Autodesk Inventor part; units mm, degrees
ref_plane "YZ Plane" through (0, 0, 0) normal (1, 0, 0) x (0, 1, 0)
ref_plane "XZ Plane" through (0, 0, 0) normal (0, 1, 0) x (-1, 0, 0)
ref_plane "XY Plane" through (0, 0, 0) normal (0, 0, 1) x (1, 0, 0)
sketch "Sketch1" plane through (0, 0, 0) normal (0, 1, 0) x (-1, 0, 0)
  line L0 (0, 0) -> (40.2, 0)
  line L1 (40.2, 0) -> (40.2, -155.2)
  line L2 (40.2, -155.2) -> (0, -155.2)
  line L3 (0, -155.2) -> (0, 0)
  line L4 (0, -20) -> (20.2, -20)
  line L5 (20.2, -20) -> (20.2, -135.2)
  line L6 (20.2, -135.2) -> (0, -135.2)
  line L7 (0, -135.2) -> (0, -20)
  line L8 (10.1, -135.2) -> (10.1, -20) construction
  line L9 (20.2, -77.6) -> (0, -77.6) construction
  circle A0 centre (10.1, -77.6) radius 3.5
  line L10 (0, -54.6) -> (20.2, -54.6) construction
  line L11 (20.2, -31.6) -> (0, -31.6) construction
  circle A1 centre (10.1, -54.6) radius 3.5
  circle A2 centre (10.1, -31.6) radius 3.5
  circle A3 centre (10.1, -100.6) radius 3.5
  circle A4 centre (10.1, -123.6) radius 3.5
  line L12 (40.2, -155.2) -> (20.2, -135.2) construction
  line L13 (30.2, -155.2) -> (30.2, 0) construction
  line L14 (20.2, -20) -> (40.2, 0) construction
  circle A5 centre (30.2, -145.2) radius 2.6
  circle A6 centre (30.2, -10) radius 2.6
  circle A7 centre (30.2, -77.6) radius 2.6
  point P0 (0, -135.2)
  dimension "d0" = 115.2
  dimension "d1" = 20.2
  dimension "d2" = 7
  dimension "d3" = 23
  dimension "d4" = 23
  dimension "d11" = 20
  dimension "d12" = 20
  dimension "d13" = 20
  dimension "d14" = 5.2
extrude "Extrusion1" add sketch "Sketch1" along normal blind 12 contours L4 L5 L6 L3
extrude "Extrusion2" add sketch "Sketch1" along normal blind 2 contours A0 | A1 | A2 | A3 | A4
extrude "Extrusion3" add sketch "Sketch1" along normal blind 19 contours L0 L1 L2 L3 L6 L5 L4
equation "\"d1\" = screwTabWidth + tolerance"
equation "\"d2\" = insertDiameter"
equation "\"d11\" = screwTabWidth"
equation "\"d12\" = screwTabWidth"
equation "\"d13\" = screwTabWidth"
equation "\"d14\" = screwDiameter + tolerance"
equation "\"d5\" = insertPadding + insertLength"
equation "\"d7\" = insertPadding"
equation "\"d9\" = insertLength + insertPadding + baseThickness"
equation "\"insertDiameter\" = 7"
equation "\"insertLength\" = 10"
equation "\"insertPadding\" = 2"
equation "\"tolerance\" = 0.2"
equation "\"cellSpacing_1\" = 1"
equation "\"screwDiameter_1\" = 5"
equation "\"baseThickness_1\" = 7"
equation "\"tabThickness_1\" = 0.8"
equation "\"batteryBoxWidth\" = 162"
equation "\"sheetMetalThickness\" = 3.175"
properties part number "CO-1-1-CellSpacerMount"
CAD build for the part. Positions are in the model's coordinates, mm. A direction names the side the tool comes from. Coordinates: 2 decimals unless noted, no trailing zeros. Write each loop counter-clockwise with the first axis right and the second up, starting at its lowest first coordinate (ties: lowest second). Pieces come first, ordered by that corner, then holes. Notation, with made-up numbers: (-16.5, -6) -> (6.5, -6) arc R15 cw to (6.5, 19) -> close; hole circle Ø10 at (81, 68). An arc over 180 degrees is marked (long way). Use CSV: the item, a comma, the result in double quotes. Start each with the question number.
Item 1: Band-saw the part on C-C, the plane x = -30.2. Write the cut outline in (y, z), plus the area to 3 significant figures.
Item 2: Band-saw the part on D-D, the plane z = -54.6. Write the cut outline in (x, y).
Item 3: Band-saw the part on A-A, the plane z = -145.2. Write the cut outline in (x, y).
Item 4: Drop flat-ended pins along their axis: P1, Ø9, axis at x = -10.1, z = -31.6, coming from the +Y side; P2, Ø4, axis at x = -30.2, z = -145.2, coming from the +Y side; P3, Ø4, axis at x = -10.1, z = -100.6, coming from the +Y side; P4, Ø3.5, axis at y = 15, z = -89.5, coming from the +X side. Give the stop position or say it passes through.
Item 5: Tool access for faces 1 (the flat face through (-5, 12, -77)), 2 (the flat face through (-20, 9, -155.2)), 3 (the flat face through (-10, 2, -32)): list every direction of +Z, -Z, +X, -X, +Y, -Y with a clear straight run to the whole face (end or side of a thin tool).
Item 6: Two-plate mould, pull along X, no slides. Class faces 4 (the cylindrical face through (-7.52, 6.93, -125.965)), 5 (the flat face through (0, 7, -79)), 6 (the cylindrical face through (-28.137, 9.367, -76.018)), 7 (the flat face through (-40.2, 9, -77)): +X half, -X half, draft (parallel to the pull), parting line (faces both ways), or undercut.
Item 7: Band-saw the part on B-B, the plane y = 9. Give the number of separate pieces and of enclosed holes in the cut face, plus the area to 3 significant figures.
Item 8: Wall check: probe 1 along Z at (x, y) = (-30.2, 10.5); probe 2 along Z at (x, y) = (-10.1, 4); probe 3 along Z at (x, y) = (-32.5, 13). Give the ranges that are in metal, low to high.
Response values:
1,outline,"(0, -155.2) -> (19, -155.2) -> (19, -147.8) -> (0, -147.8) -> close; (0, -142.6) -> (19, -142.6) -> (19, -80.2) -> (0, -80.2) -> close; (0, -75) -> (19, -75) -> (19, -12.6) -> (0, -12.6) -> close; (0, -7.4) -> (19, -7.4) -> (19, 0) -> (0, 0) -> close"
1,area,"2,650 mm2"
2,outline,"(-40.2, 0) -> (0, 0) -> (0, 12) -> (-6.6, 12) -> (-6.6, 2) -> (-13.6, 2) -> (-13.6, 12) -> (-20.2, 12) -> (-20.2, 19) -> (-40.2, 19) -> close"
3,outline,"(-40.2, 0) -> (-32.8, 0) -> (-32.8, 19) -> (-40.2, 19) -> close; (-27.6, 0) -> (0, 0) -> (0, 19) -> (-27.6, 19) -> close"
4,P1,"stops at y = 12"
4,P2,"passes through"
4,P3,"stops at y = 2"
4,P4,"stops at x = -20.2"
5,face 1,"+X, +Y"
5,face 2,"-Z, +X, -X, +Y, -Y"
5,face 3,"+Y"
6,face 4,"undercut"
6,face 5,"+X half"
6,face 6,"undercut"
6,face 7,"-X half"
7,separate pieces,"1"
7,enclosed holes,"8"
7,area,"5,980 mm2"
8,probe 1,"z = -155.2 to -147.8, -142.6 to -80.2, -75 to -12.6, -7.4 to 0"
8,probe 2,"z = -155.2 to -127.1, -120.1 to -104.1, -97.1 to -81.1, -74.1 to -58.1, -51.1 to -35.1, -28.1 to 0"
8,probe 3,"z = -155.2 to -146.41, -143.99 to -78.81, -76.39 to -11.21, -8.79 to 0"
